For this review, use the dimensioned drawing (mm, ordinates from the lowest corner) and the shaded views. A direction names the side the tool comes from. Give positions to 0.01 mm unless a question says otherwise; leave off trailing zeros. Loops run counter-clockwise (first coordinate to the right, second up) from the corner with the lowest first, then second, coordinate; pieces in that order, holes last. Notation, with made-up numbers: M -11.5,75 L 9.5,75 A34 cw 9.5,107 Z; hole C -9,21 d11. An arc over 180 degrees is marked long. Use CSV: the item, a comma, the result in double quotes. Start each with the question number.
1. Take a section at B-B, the plane x = 105. Write out the cut boundary in (y, z), and give its area (3 significant figures).
2. Tool access review of the marked faces 4 and 5: name each direction out of +Z, -Z, +X, -X, +Y, -Y from which nothing blocks a thin tool from reaching the whole face with its end or side.
3. Take a section at A-A, the plane y = 105. Write out the cut boundary in (x, z).
4. Take a section at D-D, the plane y = 63. Write out the cut boundary in (x, z) (1 decimal), and give its area (3 significant figures).
5. Take a section at C-C, the plane z = 59. State how many separate pieces and enclosed holes the cut face has, and give its area (3 significant figures).
6. The part is to be moulded in two halves that separate along Y. For the marked faces 1, 2 and 3, say which applies: pulls with the +Y half, pulls with the -Y half, needs draft (parallel to the pull), parting line crosses it, or undercut.
7. To check wall thickness, follow line 1 (Y direction, x = 137.5, z = 80.5) (1 decimal); line 2 (Y direction, x = 148.5, z = 71.5) (1 decimal); line 3 (X direction, y = 88.5, z = 29) (1 decimal). State the ranges of each line that lie inside material, in increasing order. Write a range as [from, to].
8. Insertion check: P1, Ø12, axis at y = 189.5, z = 75.5, coming from the -X side; P2, Ø8, axis at x = 181, y = 204, coming from the +Z side; P3, Ø12, axis at y = 185, z = 50.5, coming from the +X side; P4, Ø1.5, axis at y = 197, z = 50.5, coming from the -X side. Each pin has a flat end and moves straight along its axis. Give the tip position at first contact, or say it passes through.
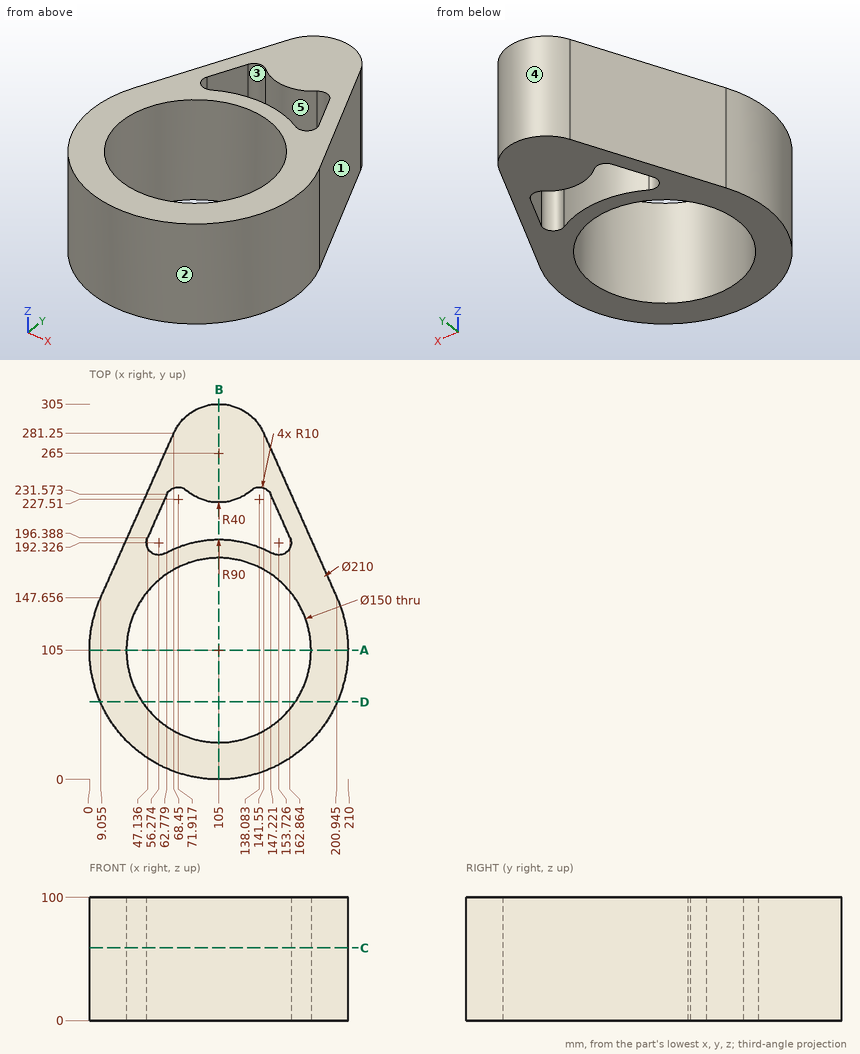
Result set:
1,outline,"M 0,0 L 30,0 L 30,100 L 0,100 Z; M 180,0 L 195,0 L 195,100 L 180,100 Z; M 225,0 L 305,0 L 305,100 L 225,100 Z"
1,area,"12,500 mm2"
2,face 4,"+Z, -Z, +Y"
2,face 5,"+Z, -Z"
3,outline,"M 0,0 L 30,0 L 30,100 L 0,100 Z; M 180,0 L 210,0 L 210,100 L 180,100 Z"
4,outline,"M 8.8,0 L 42.9,0 L 42.9,100 L 8.8,100 Z; M 167.1,0 L 201.2,0 L 201.2,100 L 167.1,100 Z"
4,area,"6,820 mm2"
5,separate pieces,"1"
5,enclosed holes,"2"
5,area,"23,000 mm2"
6,face 1,"pulls with the +Y half"
6,face 2,"parting line crosses it"
6,face 3,"undercut"
7,line 1,"[5.2, 37.4], [172.6, 188.9], [237.5, 288.3]"
7,line 2,"[9.4, 43.9], [166.1, 183.8], [228.7, 265.6]"
7,line 3,"[1.3, 31.8], [178.2, 208.7]"
8,P1,"x = 24.99"
8,P2,"through"
8,P3,"x = 187.01"
8,P4,"x = 30.66"
